```python
from build123d import *

# Parameters (mm, degrees)
F0_R          = 88.9
F1_DEPTH      = 12.7
F2_R          = 88.9
F2_R_2        = 82.55
F2_R_3        = 6.35
F3_DEPTH      = 25.4
F5_DEPTH      = 25.4
F7_DEPTH      = 25.4
F8_W          = 12.7
F8_H          = 1.27
F9_DEPTH      = 19.05
F10_W         = 19.05
F10_H         = 25.4
F11_DEPTH     = 88.901
F12_T1_DEPTH  = 19.05
F12_T6_ANGLE  = 25.274429264
F12_T12_ANGLE = 25.274429264
F12_T19_ANGLE = 25.274429264
F12_T23_DEPTH = 24.7827133537
F12_T30_ANGLE = 25.274429264
F12_T34_DEPTH = 24.7827133537
F12_T41_DEPTH = 29.3229812516
F12_T45_ANGLE = 25.274429264
F12_T52_ANGLE = 25.274429264
F12_T56_DEPTH = 29.3229812516
F14_DEPTH     = 25.4
F16_DEPTH     = 38.1
F20_DEPTH     = 25.4


# Not quite as in the source:
# - a fillet or chamfer that OpenCascade refuses, or shapes differently, is made with other operations: its cross-section is extruded or revolved along the edge and cut away or added


with BuildPart() as f1:
    # F0 (on Front) → F1 (new body)
    with BuildSketch(Plane.XZ):
        Circle(F0_R)
    extrude(amount=F1_DEPTH)

    # F2 (on face) → F3 (join)
    with BuildSketch(Plane.XZ.offset(12.7)):
        Circle(F2_R)
        Circle(F2_R_2, mode=Mode.SUBTRACT)
        Circle(F2_R_3)
    extrude(amount=F3_DEPTH)

    # F4 (on face) → F5 (cut)
    with BuildSketch(Plane.XZ.offset(38.1)):
        with BuildLine():
            Line((-34.9300524425, 74.7956812681), (-38.9724939218, 79.9021571518))
            ThreePointArc((-38.9724939218, 79.9021571518), (-51.1040456605, 72.7432919047), (-61.9525410202, 63.7580791833))
            Line((-61.9525410202, 63.7580791833), (-58.1372414147, 58.6051504621))
            ThreePointArc((-58.1372414147, 58.6051504621), (-47.2325482948, 67.7022073612), (-34.9300524425, 74.7956812681))
        make_face()
    extrude(amount=-F5_DEPTH, mode=Mode.SUBTRACT)

    # F6 (on face) → F7 (join)
    with BuildSketch(Plane.XZ.offset(12.7)):
        with BuildLine():
            ThreePointArc((-33.5668462981, 63.0071964846), (-35.8100364522, 66.042382708), (-39.3699048248, 64.7887501268))
            Line((-39.3699048248, 64.7887501268), (-34.1137877714, 61.2256428423))
            ThreePointArc((-34.1137877714, 61.2256428423), (-33.7066600747, 62.0753866387), (-33.5668462981, 63.0071964846))
        make_face()
        with BuildLine():
            Line((-34.1137877714, 61.2256428423), (-39.3699048248, 64.7887501268))
            ThreePointArc((-39.3699048248, 64.7887501268), (-38.5233999404, 60.3791379579), (-34.1137877714, 61.2256428423))
        make_face()
    extrude(amount=F7_DEPTH)

    # F8 (on face) → F9 (cut)
    with BuildSketch(Plane.XZ.offset(38.1)):
        with Locations((0, 0.635)):
            Rectangle(F8_W, F8_H)
        with Locations((0, -0.635)):
            Rectangle(F8_W, F8_H)
    extrude(amount=-F9_DEPTH, mode=Mode.SUBTRACT)

    # F10 (on Right) → F11 (cut, through all)
    with BuildSketch(Plane.YZ):
        with Locations((-22.225, -24.1626900017)):
            Rectangle(F10_W, F10_H)
    extrude(amount=-F11_DEPTH, mode=Mode.SUBTRACT)

    # F12: fillet of radius 2.54 on 4 edges, made by hand

    # F12_s2 → F12_t1 (cut)
    with BuildSketch(Plane.XZ.offset(12.7)):
        with BuildLine():
            ThreePointArc((-88.4242248071, -9.1851220606), (-87.5985568369, -10.8092447226), (-85.897818384, -11.4626900017))
            Line((-85.897818384, -11.4626900017), (-88.1579079716, -11.4626900017))
            ThreePointArc((-88.1579079716, -11.4626900017), (-88.2984101391, -10.3247647385), (-88.4242248071, -9.1851220606))
        make_face()
        with BuildLine():
            ThreePointArc((-79.1073144645, -40.5615926488), (-79.0145016969, -38.078305753), (-76.8471054798, -36.8626900017))
            Line((-76.8471054798, -36.8626900017), (-80.8971698259, -36.8626900017))
            ThreePointArc((-80.8971698259, -36.8626900017), (-80.0236166295, -38.7224841861), (-79.1073144645, -40.5615926488))
        make_face()
    extrude(amount=F12_T1_DEPTH, mode=Mode.SUBTRACT)


with BuildPart() as f12_tool4:
    # F12_s5 → F12_t6 (revolve)
    with BuildSketch(Plane(origin=(0, 0, 0), x_dir=(0, 1, 0), z_dir=(0.478540272, 0, -0.8780656058))):
        with BuildLine():
            ThreePointArc((-10.16, -88.9), (-11.9560512242, -88.1560512242), (-12.7, -86.36))
            Line((-12.7, -86.36), (-12.7, -88.9))
            Line((-12.7, -88.9), (-10.16, -88.9))
        make_face()
    revolve(axis=Axis((0, -12.7, 0), (0, 1, 0)), revolution_arc=F12_T6_ANGLE)

    split(bisect_by=Plane.XY.offset(-11.4626900017), keep=Keep.BOTTOM)

    split(bisect_by=Plane.XY.offset(-36.8626900017), keep=Keep.TOP)


with BuildPart() as f1_1:
    add(f1.part)

    # F12_t3: cut F12_tool4
    add(f12_tool4.part, mode=Mode.SUBTRACT)


with BuildPart() as f12_tool10:
    # F12_s11 → F12_t12 (revolve)
    with BuildSketch(Plane(origin=(0, 0, 0), x_dir=(0, 1, 0), z_dir=(0.478540272, 0, -0.8780656058))):
        with BuildLine():
            ThreePointArc((-34.29, -88.9), (-32.4939487758, -88.1560512242), (-31.75, -86.36))
            Line((-31.75, -86.36), (-31.75, -88.9))
            Line((-31.75, -88.9), (-34.29, -88.9))
        make_face()
    revolve(axis=Axis((0, -31.75, 0), (0, 1, 0)), revolution_arc=F12_T12_ANGLE)

    split(bisect_by=Plane.XY.offset(-36.8626900017), keep=Keep.TOP)

    split(bisect_by=Plane.XY.offset(-11.4626900017), keep=Keep.BOTTOM)


with BuildPart() as f1_2:
    add(f1_1.part)

    # F12_t9: cut F12_tool10
    add(f12_tool10.part, mode=Mode.SUBTRACT)


with BuildPart() as f12_tool17:
    # F12_s18 → F12_t19 (revolve)
    with BuildSketch(Plane(origin=(0, 0, 0), x_dir=(0, 1, 0), z_dir=(0.478540272, 0, -0.8780656058))):
        with BuildLine():
            ThreePointArc((-34.29, -88.9), (-32.4939487758, -88.1560512242), (-31.75, -86.36))
            Line((-31.75, -86.36), (-31.75, -88.9))
            Line((-31.75, -88.9), (-34.29, -88.9))
        make_face()
    revolve(axis=Axis((0, -31.75, 0), (0, 1, 0)), revolution_arc=F12_T19_ANGLE)

    split(bisect_by=Plane.XY.offset(-11.4626900017), keep=Keep.TOP)


with BuildPart() as f12_tool21:
    # F12_s22 → F12_t23 (new body)
    with BuildSketch(Plane.XZ.offset(37.4827133537)):
        with BuildLine():
            ThreePointArc((-88.4242248071, -9.1851220606), (-87.5985568369, -10.8092447226), (-85.897818384, -11.4626900017))
            Line((-85.897818384, -11.4626900017), (-88.1579079716, -11.4626900017))
            ThreePointArc((-88.1579079716, -11.4626900017), (-88.2984101391, -10.3247647385), (-88.4242248071, -9.1851220606))
        make_face()
    extrude(amount=-F12_T23_DEPTH)

    split(bisect_by=Plane.XZ.offset(31.75), keep=Keep.TOP)


with BuildPart() as f12_tool17_1:
    add(f12_tool17.part)

    # F12_t25: intersect F12_tool21
    add(f12_tool21.part, mode=Mode.INTERSECT)


with BuildPart() as f1_3:
    add(f1_2.part)

    # F12_t15: cut F12_tool17
    add(f12_tool17_1.part, mode=Mode.SUBTRACT)


with BuildPart() as f12_tool28:
    # F12_s29 → F12_t30 (revolve)
    with BuildSketch(Plane(origin=(0, 0, 0), x_dir=(0, 1, 0), z_dir=(0.478540272, 0, -0.8780656058))):
        with BuildLine():
            ThreePointArc((-10.16, -88.9), (-11.9560512242, -88.1560512242), (-12.7, -86.36))
            Line((-12.7, -86.36), (-12.7, -88.9))
            Line((-12.7, -88.9), (-10.16, -88.9))
        make_face()
    revolve(axis=Axis((0, -12.7, 0), (0, 1, 0)), revolution_arc=F12_T30_ANGLE)

    split(bisect_by=Plane.XY.offset(-11.4626900017), keep=Keep.TOP)


with BuildPart() as f12_tool32:
    # F12_s33 → F12_t34 (new body)
    with BuildSketch(Plane.XZ.offset(31.75)):
        with BuildLine():
            ThreePointArc((-88.4242248071, -9.1851220606), (-87.5985568369, -10.8092447226), (-85.897818384, -11.4626900017))
            Line((-85.897818384, -11.4626900017), (-88.1579079716, -11.4626900017))
            ThreePointArc((-88.1579079716, -11.4626900017), (-88.2984101391, -10.3247647385), (-88.4242248071, -9.1851220606))
        make_face()
    extrude(amount=-F12_T34_DEPTH)

    split(bisect_by=Plane.XZ.offset(12.7), keep=Keep.BOTTOM)


with BuildPart() as f12_tool28_1:
    add(f12_tool28.part)

    # F12_t36: intersect F12_tool32
    add(f12_tool32.part, mode=Mode.INTERSECT)


with BuildPart() as f1_4:
    add(f1_3.part)

    # F12_t26: cut F12_tool28
    add(f12_tool28_1.part, mode=Mode.SUBTRACT)


with BuildPart() as f12_tool39:
    # F12_s40 → F12_t41 (new body)
    with BuildSketch(Plane.XZ.offset(31.75)):
        with BuildLine():
            ThreePointArc((-79.1073144645, -40.5615926488), (-79.0145016969, -38.078305753), (-76.8471054798, -36.8626900017))
            Line((-76.8471054798, -36.8626900017), (-80.8971698259, -36.8626900017))
            ThreePointArc((-80.8971698259, -36.8626900017), (-80.0236166295, -38.7224841861), (-79.1073144645, -40.5615926488))
        make_face()
    extrude(amount=-F12_T41_DEPTH)

    split(bisect_by=Plane.XZ.offset(12.7), keep=Keep.BOTTOM)


with BuildPart() as f12_tool43:
    # F12_s44 → F12_t45 (revolve)
    with BuildSketch(Plane(origin=(0, 0, 0), x_dir=(0, 1, 0), z_dir=(0.478540272, 0, -0.8780656058))):
        with BuildLine():
            ThreePointArc((-10.16, -88.9), (-11.9560512242, -88.1560512242), (-12.7, -86.36))
            Line((-12.7, -86.36), (-12.7, -88.9))
            Line((-12.7, -88.9), (-10.16, -88.9))
        make_face()
    revolve(axis=Axis((0, -12.7, 0), (0, 1, 0)), revolution_arc=F12_T45_ANGLE)

    split(bisect_by=Plane.XY.offset(-36.8626900017), keep=Keep.BOTTOM)


with BuildPart() as f12_tool39_1:
    add(f12_tool39.part)

    # F12_t47: intersect F12_tool43
    add(f12_tool43.part, mode=Mode.INTERSECT)


with BuildPart() as f1_5:
    add(f1_4.part)

    # F12_t37: cut F12_tool39
    add(f12_tool39_1.part, mode=Mode.SUBTRACT)


with BuildPart() as f12_tool50:
    # F12_s51 → F12_t52 (revolve)
    with BuildSketch(Plane(origin=(0, 0, 0), x_dir=(0, 1, 0), z_dir=(0.478540272, 0, -0.8780656058))):
        with BuildLine():
            ThreePointArc((-34.29, -88.9), (-32.4939487758, -88.1560512242), (-31.75, -86.36))
            Line((-31.75, -86.36), (-31.75, -88.9))
            Line((-31.75, -88.9), (-34.29, -88.9))
        make_face()
    revolve(axis=Axis((0, -31.75, 0), (0, 1, 0)), revolution_arc=F12_T52_ANGLE)

    split(bisect_by=Plane.XY.offset(-36.8626900017), keep=Keep.BOTTOM)


with BuildPart() as f12_tool54:
    # F12_s55 → F12_t56 (new body)
    with BuildSketch(Plane.XZ.offset(42.0229812516)):
        with BuildLine():
            ThreePointArc((-79.1073144645, -40.5615926488), (-79.0145016969, -38.078305753), (-76.8471054798, -36.8626900017))
            Line((-76.8471054798, -36.8626900017), (-80.8971698259, -36.8626900017))
            ThreePointArc((-80.8971698259, -36.8626900017), (-80.0236166295, -38.7224841861), (-79.1073144645, -40.5615926488))
        make_face()
    extrude(amount=-F12_T56_DEPTH)

    split(bisect_by=Plane.XZ.offset(31.75), keep=Keep.TOP)


with BuildPart() as f12_tool50_1:
    add(f12_tool50.part)

    # F12_t58: intersect F12_tool54
    add(f12_tool54.part, mode=Mode.INTERSECT)


with BuildPart() as f1_6:
    add(f1_5.part)

    # F12_t48: cut F12_tool50
    add(f12_tool50_1.part, mode=Mode.SUBTRACT)

    # F13 (on face) → F14 (cut)
    with BuildSketch(Plane.XZ.offset(38.1)):
        with BuildLine():
            ThreePointArc((-34.9300524425, 74.7956812681), (44.3341102926, 69.6346836323), (82.55, 0))
            ThreePointArc((82.55, 0), (-31.7432923719, -76.2027944986), (-58.1372414147, 58.6051504621))
            Line((-58.1372414147, 58.6051504621), (-60.0455804339, 61.1825456757))
            ThreePointArc((-60.0455804339, 61.1825456757), (-33.1765598149, -79.0448701931), (85.725, 0))
            ThreePointArc((85.725, 0), (45.721772873, 72.5141028376), (-36.9532177975, 77.3513756788))
            Line((-36.9532177975, 77.3513756788), (-34.9300524425, 74.7956812681))
        make_face()
    extrude(amount=-F14_DEPTH, mode=Mode.SUBTRACT)

    # F15 (on face) → F16 (join)
    with BuildSketch(Plane(origin=(0, 0, 0), x_dir=(-1, 0, 0), z_dir=(0, 1, 0))):
        with BuildLine():
            Line((-125.723585695, 0), (-62.8617928475, -62.8617928475))
            ThreePointArc((-62.8617928475, -62.8617928475), (-87.5758152323, -15.286810864), (-80.4411250184, 37.8475283972))
            ThreePointArc((-80.4411250184, 37.8475283972), (-98.9019872856, 13.9221865314), (-125.723585695, 0))
        make_face()
        with BuildLine():
            ThreePointArc((37.8475283972, -80.4411250184), (19.3906418907, -86.7595124875), (0, -88.9))
            ThreePointArc((0, -88.9), (-34.0205571373, -82.1328904403), (-62.8617928475, -62.8617928475))
            Line((-62.8617928475, -62.8617928475), (0, -125.723585695))
            ThreePointArc((0, -125.723585695), (13.9221865314, -98.9019872856), (37.8475283972, -80.4411250184))
        make_face()
    extrude(amount=-F16_DEPTH)

    # F19 (on face) → F20 (cut)
    with BuildSketch(Plane(origin=(-61.6045569905, 0, 61.6045569905), x_dir=(0, -1, 0), z_dir=(-0.7071067812, 0, 0.7071067812))):
        Polygon((25.1616425812, -3.5754330456), (17.159935087, -3.5754330456), (17.159935087, -10.567618534), (11.9749652222, -10.567618534), (21.1607888341, -15.9158930182), (30.4591618478, -10.567618534), (25.1616425812, -10.567618534), align=None)
    extrude(amount=F20_DEPTH, mode=Mode.SUBTRACT)


solid = f1_6.part
```
Check sheet for the modelled part. Datum: model origin and axes. Units: mm. A direction names the side the tool comes from. Give positions to 0.01 mm unless a question says otherwise; leave off trailing zeros. Loops run counter-clockwise (first coordinate to the right, second up) from the corner with the lowest first, then second, coordinate; pieces in that order, holes last. Notation, with made-up numbers: M 56,27.25 L 86,27.25 A20 ccw 86,59.25 Z; hole C 0,34.5 d9. An arc over 180 degrees is marked long. Answer in a Markdown table with one row per item.
1) Mould release check, pull along X, two halves, no side actions. Record for faces 1 (the face through (0, -38.1, -3)), 2 (the face through (-61.15, -10.32, 64.53)), 3 (the face through (0, -29, 1.27)), 4 (the face through (80.812, -25.578, -28.604)): released by +X, released by -X, zero draft, split by the parting line, or undercut.
Solutions:
| item | result |
|---|---|
| face 1 | zero draft |
| face 2 | split by the parting line |
| face 3 | undercut |
| face 4 | undercut |
2) Cross-section at C-C (y = -7). Enter the section's corners in (x, z), plus the area to 3 significant figures.
Solutions:
| item | result |
|---|---|
| outline | M -37.85,-80.44 A70.05 cw 0,-125.72 L 125.72,0 A70.05 cw 80.44,37.85 A88.9 ccw long Z |
| area | 27,300 mm^2 |
3) Tool access check on faces 5 (the face through (-82.4, -31.75, -24.2)), 6 (the face through (0, -29, -1.27)), 7 (the face through (-70.88, -26.78, 52.94)). Record the directions out of +Z, -Z, +X, -X, +Y, -Y that give a thin tool (end or side, any length) a straight path to the whole face; none if there is none.
Solutions:
| item | result |
|---|---|
| face 5 | -X |
| face 6 | -Y |
| face 7 | none |
4) Depth check by flat-ended pin: pin 1 (4 mm diameter, centred on x = -25, y = -30.5, fed in from +Z); pin 2 (3 mm diameter, centred on x = 38, y = -28.5, fed in from +Z); pin 3 (1 mm diameter, centred on y = -19.5, z = -75, fed in from -X). Enter the tip coordinate at first touch or a pass-through.
Solutions:
| item | result |
|---|---|
| pin 1 | stops at z = 85.87 |
| pin 2 | stops at z = 81.06 |
| pin 3 | stops at x = -48.51 |
5) Cross-section at D-D (z = 73). Enter the section's corners in (x, y), plus the area to 3 significant figures.
Solutions:
| item | result |
|---|---|
| outline | M -50.74,-12.7 L 44.94,-12.7 L 44.94,-38.1 L 50.74,-38.1 L 50.74,0 L -50.74,0 Z |
| area | 1,440 mm^2 |
6) Cross-section at B-B (z = -50.5). Enter the section's corners in (x, y), plus the area to 3 significant figures.
Solutions:
| item | result |
|---|---|
| outline | M -73.16,-38.1 L -69.27,-38.1 L -69.27,-12.7 L 69.27,-12.7 L 69.27,-38.1 L 75.22,-38.1 L 75.22,0 L -73.16,0 Z |
| area | 2,130 mm^2 |
7) Cross-section at A-A (x = 25.5). Enter the section's corners in (y, z).
Solutions:
| item | result |
|---|---|
| outline | M -38.1,-100.22 L 0,-100.22 L 0,85.16 L -38.1,85.16 L -38.1,81.84 L -12.7,81.84 L -12.7,-81.84 L -38.1,-81.84 Z |
8) Thickness scan on line 1 (Y direction, x = 54, z = -40.5); line 2 (Z direction, x = -36.5, y = -31.5); line 3 (Z direction, x = 74.5, y = -31.5). Record the ranges inside material, lowest first.
Solutions:
| item | result |
|---|---|
| line 1 | y = -12.7 to 0 |
| line 2 | z = -81.09 to -77.57, 59.84 to 66.17, 77.57 to 81.06 |
| line 3 | z = -51.22 to -42.41, 42.41 to 48.51 |
